```python
from build123d import *

# Parameters (mm, degrees)
F0_W     = 2500
F0_H     = 1400
F1_DEPTH = 25


with BuildPart() as f1:
    # F0 (on Front) → F1 (new body)
    with BuildSketch(Plane.XZ):
        with Locations((1250, 700)):
            Rectangle(F0_W, F0_H)
        Polygon((40, 1337.2182471161), (40, 1360), (81.7665469538, 1360), (2460, 1360), (2460, 1040), (2460, 1000), (2460, 62.7817528839), (2460, 40), (2418.2334530462, 40), (40, 40), (40, 1000), (40, 1040), align=None, mode=Mode.SUBTRACT)
        Polygon((2460, 62.7817528839), (741.7665469538, 1000), (658.2334530462, 1000), (2418.2334530462, 40), (2460, 40), align=None)
        Polygon((2460, 1040), (668.4332136205, 1040), (741.7665469538, 1000), (2460, 1000), align=None)
        Polygon((81.7665469538, 1360), (40, 1360), (40, 1337.2182471161), (584.9001197129, 1040), (668.4332136205, 1040), align=None)
        Polygon((584.9001197129, 1040), (40, 1040), (40, 1000), (658.2334530462, 1000), align=None)
        Polygon((741.7665469538, 1000), (668.4332136205, 1040), (584.9001197129, 1040), (658.2334530462, 1000), align=None)
    extrude(amount=F1_DEPTH)


solid = f1.part
```
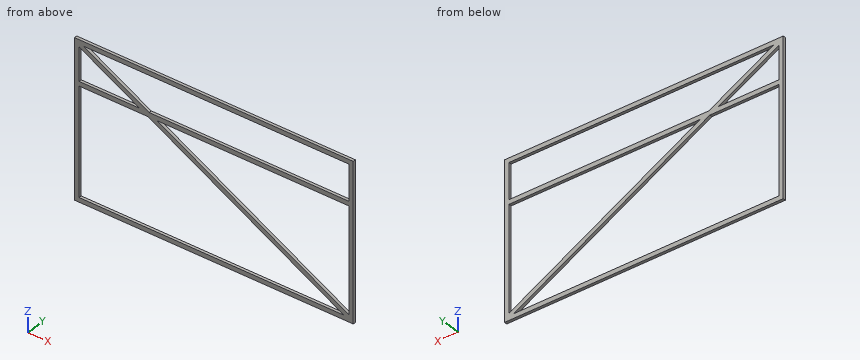
Here's how the part is built. I have some questions about the finished solid (model axes, mm). Coordinates: 2 decimals unless noted, no trailing zeros. Loops run counter-clockwise (first coordinate to the right, second up) from the corner with the lowest first, then second, coordinate; pieces in that order, holes last. Notation, with made-up numbers: (80, -23.75) - (114, -23.75) arc R30 cw to (114, 11.25) - close; hole circle Ø6 at (-31.5, 58.5). An arc over 180 degrees is marked (long way). Return JSON: item names as keys, results as strings. Group by question number.
Item 1: If we section it at B-B on z = 781.5: Write out the boundary of the cut face in (x, y).
Item 2: I need wall thicknesses on line 1 (Z direction, x = 1732, y = -23.75); line 2 (X direction, y = -12, z = 1212); line 3 (X direction, y = -9.25, z = 1307). Which ranges of each line are inside material? Lowest first, please. Write a range as from..to.
Item 3: If we section it at A-A on y = -7.25: Write out the boundary of the cut face in (x, z).
Item 4: If we section it at C-C on x = 801.5: Write out the boundary of the cut face in (y, z).
Calculated:
{
 "1": {"outline": "(0, -25) - (40, -25) - (40, 0) - (0, 0) - close; (1058.82, -25) - (1142.35, -25) - (1142.35, 0) - (1058.82, 0) - close; (2460, -25) - (2500, -25) - (2500, 0) - (2460, 0) - close"},
 "2": {"line 1": "z = 0..40, 414.31..459.87, 1000..1040, 1360..1400", "line 2": "x = 0..40, 269.57..353.1, 2460..2500", "line 3": "x = 0..40, 95.4..178.93, 2460..2500"},
 "3": {"outline": "(0, 0) - (2500, 0) - (2500, 1400) - (0, 1400) - close; hole (40, 40) - (2418.23, 40) - (658.23, 1000) - (40, 1000) - close; hole (40, 1040) - (584.9, 1040) - (40, 1337.22) - close; hole (81.77, 1360) - (668.43, 1040) - (2460, 1040) - (2460, 1360) - close; hole (741.77, 1000) - (2460, 62.78) - (2460, 1000) - close"},
 "4": {"outline": "(-25, 0) - (0, 0) - (0, 40) - (-25, 40) - close; (-25, 921.85) - (0, 921.85) - (0, 967.42) - (-25, 967.42) - close; (-25, 1000) - (0, 1000) - (0, 1040) - (-25, 1040) - close; (-25, 1360) - (0, 1360) - (0, 1400) - (-25, 1400) - close"}
}
